```python
from build123d import *

# Parameters (mm, degrees)
SKETCH_R    = 2.5
PAD_DEPTH   = 6.7
FILLET_R    = 3
FILLET001_R = 3


with BuildPart() as part:
    # Sketch → Pad (new body)
    with BuildSketch(Plane.XY):
        Polygon((0, 0), (6, 0), (6, -8.17137), (31, -8.17137), (31, 0), (37, 0), (37, 9), (0, 9), align=None)
        with Locations((6.5, 5)):
            Circle(SKETCH_R, mode=Mode.SUBTRACT)
        with Locations((30.5, 5)):
            Circle(SKETCH_R, mode=Mode.SUBTRACT)
    extrude(amount=PAD_DEPTH)

    # Fillet
    fillet_edges = [part.edges().sort_by_distance(p)[0] for p in [
        (37, 9, 3.35),
    ]]
    fillet(fillet_edges, radius=FILLET_R)

    # Fillet001
    fillet001_edges = [part.edges().sort_by_distance(p)[0] for p in [
        (0, 9, 3.35),
    ]]
    fillet(fillet001_edges, radius=FILLET001_R)


solid = part.part
```
Work out the finished part from the listing and answer in its coordinate system (mm). A direction names the side the tool comes from. Coordinates: 2 decimals unless noted, no trailing zeros. Order: outer loops, then holes, each group sorted by start corner. A loop starts at its lowest first (then second) coordinate and runs counter-clockwise, first axis right, second up. Notation, with made-up numbers: (-3, 66) - (56, 66) arc R30 ccw to (56, 103) - close; hole circle Ø2 at (12, 53.25). An arc over 180 degrees is marked (long way). Answer as a JSON object with one key per item and string values.
1. A tool of negligible diameter and unlimited length cuts with its end or side. For faces 5 (the face through (18, 1, 6.7)), 6 (the face through (6, -4, 3)), 7 (the face through (34, 0, 3)), from which of +Z, -Z, +X, -X, +Y, -Y can it reach the whole face along a straight path? Write none if from no direction.
Output values:
{"face 5": "+Z, +X, -X, +Y, -Y", "face 6": "+Z, -Z, -X, -Y", "face 7": "+Z, -Z, +X, -Y"}
2. Find section D-D on y = -4.5. Determine the outline of the cut face in (x, z).
Output values:
{"outline": "(6, 0) - (31, 0) - (31, 6.7) - (6, 6.7) - close"}
3. Find section A-A on z = 3.75. Determine the outline of the cut face in (x, y), plus the area to 3 significant figures.
Output values:
{"outline": "(0, 0) - (6, 0) - (6, -8.17) - (31, -8.17) - (31, 0) - (37, 0) - (37, 6) arc R3 ccw to (34, 9) - (3, 9) arc R3 ccw to (0, 6) - close; hole circle Ø5 at (6.5, 5); hole circle Ø5 at (30.5, 5)", "area": "494 mm²"}
4. Consider line 1 (Y direction, x = 6.5, z = 5); line 2 (X direction, y = 4.25, z = 3.25); line 3 (X direction, y = -6, z = 4.5). Determine where each line is inside the solid, lowest interval first.
Output values:
{"line 1": "y = -8.17 to 2.5, 7.5 to 9", "line 2": "x = 0 to 4.12, 8.88 to 28.12, 32.88 to 37", "line 3": "x = 6 to 31"}
5. Each of these flat-tipped pins is pushed along its axis until it touches: P1, Ø4, axis at x = 6.5, y = 5, coming from the +Z side; P2, Ø3, axis at x = 1.5, z = 2.5, coming from the -Y side; P3, Ø2, axis at y = -3, z = 2.5, coming from the +X side; P4, Ø1.5, axis at y = -2, z = 3, coming from the -X side. Where does it stop, or does it pass through?
Output values:
{"P1": "passes through", "P2": "stops at y = 0", "P3": "stops at x = 31", "P4": "stops at x = 6"}
6. Find section C-C on y = 5. Determine the outline of the cut face in (x, z).
Output values:
{"outline": "(0, 0) - (4, 0) - (4, 6.7) - (0, 6.7) - close; (9, 0) - (28, 0) - (28, 6.7) - (9, 6.7) - close; (33, 0) - (37, 0) - (37, 6.7) - (33, 6.7) - close"}
7. The mould has two halves that part along Y. Classify faces 1 (the face through (36.1, 8.14, 3.4)), 2 (the face through (31, -4, 3)), 3 (the face through (18, -8.171, 3)), 4 (the face through (29, 7, 3)): +Y half, -Y half, draft (parallel to the pull), parting line (faces both ways), or undercut.
Output values:
{"face 1": "+Y half", "face 2": "draft", "face 3": "-Y half", "face 4": "undercut"}
8. Find section B-B on x = 30.5. Determine the outline of the cut face in (y, z).
Output values:
{"outline": "(-8.17, 0) - (2.5, 0) - (2.5, 6.7) - (-8.17, 6.7) - close; (7.5, 0) - (9, 0) - (9, 6.7) - (7.5, 6.7) - close"}
